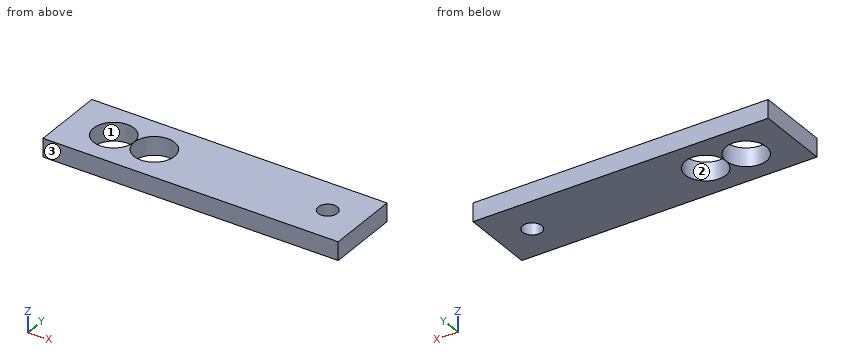
```python
from build123d import *

# Parameters (mm, degrees)
ESBO_O1_W             = 51
ESBO_O1_H             = 12.7
FLANGE_BASE1_DEPTH    = 3.18
ESBO_O2_R             = 3.5
ESBO_O2_R_2           = 1.65
CORTE_EXTRUS_O1_DEPTH = 10


# Sheet-metal steps are written as plain solids
with BuildPart() as part:
    # Esboço1 → Flange-base1 (new body)
    with BuildSketch(Plane.XY):
        Rectangle(ESBO_O1_W, ESBO_O1_H)
    extrude(amount=-FLANGE_BASE1_DEPTH)

    # Esboço2 → Corte-extrusão1 (cut)
    with BuildSketch(Plane(origin=(0, 0, -3.18), x_dir=(-1, 0, 0), z_dir=(0, 0, -1))):
        with Locations((17.485, 0)):
            Circle(ESBO_O2_R)
        with Locations((-19.4825, 0)):
            Circle(ESBO_O2_R_2)
        with Locations((10.484, 0)):
            Circle(ESBO_O2_R)
    extrude(amount=-CORTE_EXTRUS_O1_DEPTH, mode=Mode.SUBTRACT)


solid = part.part
```
Geometry: final body of the model. Coordinates: model frame, mm. Face numbers are marked on the shaded views. Round coordinates to 2 decimals unless told otherwise and drop trailing zeros. Loops run counter-clockwise (first coordinate to the right, second up) from the corner with the lowest first, then second, coordinate; pieces in that order, holes last.
Item 1: Section A-A, the plane z = -2.05. State how many separate pieces and enclosed holes the cut face has, plus the area to 3 significant figures.
Checked values:
separate pieces: 1
enclosed holes: 3
area: 562 mm2
Item 2: Contact query for a flat-ended pin moving along its axis: P1, Ø6.5, axis at x = -17.485, y = 0, coming from the -Z side. Output: stop coordinate, or through.
Checked values:
P1: passes through
Item 3: Mould query, pull axis X, two halves, no side actions, for the marked faces 1, 2 and 3. Classes: released by +X, released by -X, zero draft, split by the parting line, or undercut.
Checked values:
face 1: undercut
face 2: undercut
face 3: zero draft
Item 4: Section C-C, the plane x = 20.5. Output: boundary loops of the cut face in (y, z), plus the area to 3 significant figures.
Checked values:
outline: (-6.35, -3.18) - (-1.3, -3.18) - (-1.3, 0) - (-6.35, 0) - close; (1.3, -3.18) - (6.35, -3.18) - (6.35, 0) - (1.3, 0) - close
area: 32.1 mm2
Item 5: Line query: L1, parallel to X at y = -1.25, z = -2.25; L2, parallel to X at y = 2, z = -3; L3, parallel to Y at x = -9.5, z = -2.35. Output: solid intervals per line, ascending.
Checked values:
L1: x = -25.5 to -20.75, -14.22 to -13.75, -7.21 to 18.41, 20.56 to 25.5
L2: x = -25.5 to -20.36, -14.61 to -13.36, -7.61 to 25.5
L3: y = -6.35 to -3.36, 3.36 to 6.35
